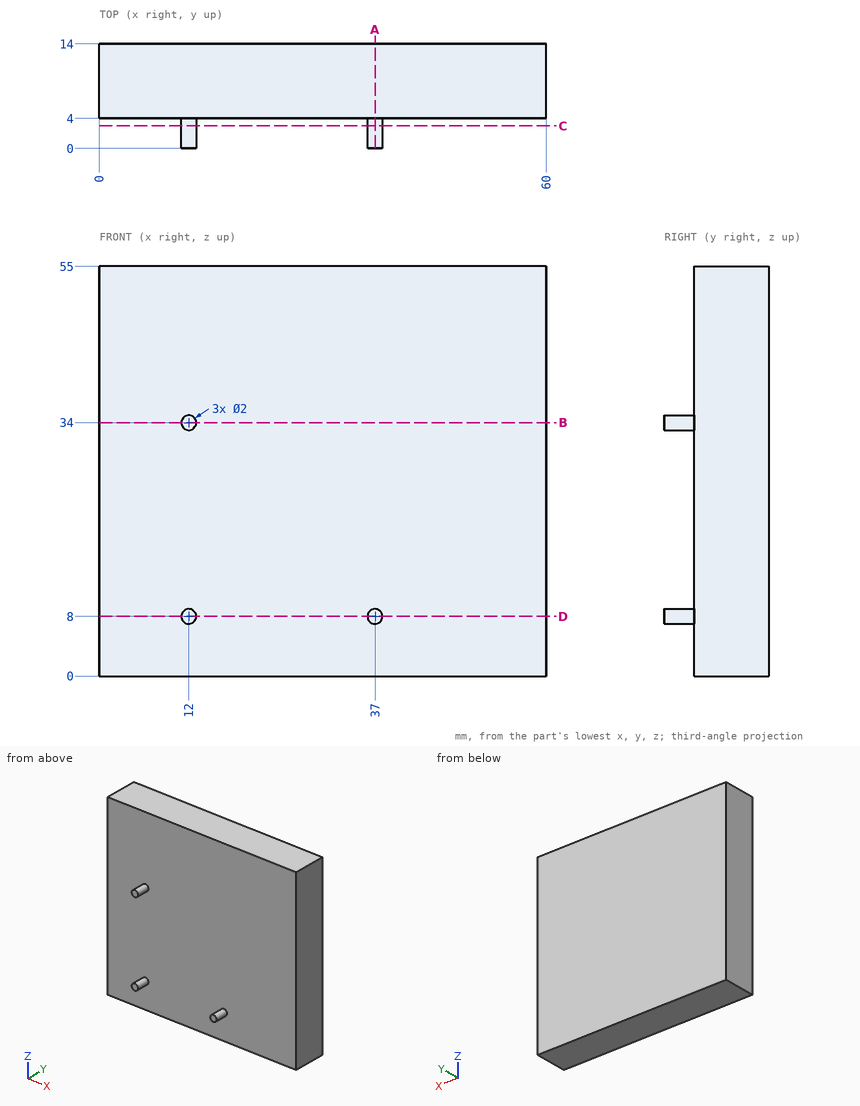
The figure shows three views and two pictorial views of one solid part (mm, origin at its lowest corner). Answer the questions. Give positions to 0.01 mm unless a question says otherwise; leave off trailing zeros. Write each loop counter-clockwise with the first axis right and the second up, starting at its lowest first coordinate (ties: lowest second). Pieces come first, ordered by that corner, then holes. Notation, with made-up numbers: (57, 88.5) -> (114, 88.5) arc R5 cw to (114, 93.5) -> close; hole circle Ø10 at (62.5, 46). An arc over 180 degrees is marked (long way). Use one line per item in the form item = value.
1) Section D-D on z = 8 is taken. Write down the section's boundary in (x, y), plus the area to 3 significant figures.
Result:
outline = (0, 4) -> (11, 4) -> (11, 0) -> (13, 0) -> (13, 4) -> (36, 4) -> (36, 0) -> (38, 0) -> (38, 4) -> (60, 4) -> (60, 14) -> (0, 14) -> close
area = 616 mm²
2) Each of these flat-tipped pins is pushed along its axis until it touches: P1, Ø8, axis at x = 47.5, y = 5.5, coming from the -Z side; P2, Ø4, axis at x = 22.5, z = 19, coming from the -Y side. Where does it stop, or does it pass through?
Result:
P1 = 0
P2 = 4
3) Section B-B on z = 34 is taken. Write down the section's boundary in (x, y), plus the area to 3 significant figures.
Result:
outline = (0, 4) -> (11, 4) -> (11, 0) -> (13, 0) -> (13, 4) -> (60, 4) -> (60, 14) -> (0, 14) -> close
area = 608 mm²
4) Section A-A on x = 37 is taken. Write down the section's boundary in (y, z).
Result:
outline = (0, 7) -> (4, 7) -> (4, 0) -> (14, 0) -> (14, 55) -> (4, 55) -> (4, 9) -> (0, 9) -> close
5) Section C-C on y = 3 is taken. Write down the section's boundary in (x, z).
Result:
outline = circle Ø2 at (12, 8); circle Ø2 at (12, 34); circle Ø2 at (37, 8)
6) A straight line is drawn through the part: probe 1 along Y at (x, z) = (8, 26). Find the intervals that lie inside material, in ascending order.
Result:
probe_1 = 4 to 14
